Work out the finished part from the listing and answer in its coordinate system (mm). A direction names the side the tool comes from. Give positions to 0.01 mm unless a question says otherwise; leave off trailing zeros. Loops run counter-clockwise (first coordinate to the right, second up) from the corner with the lowest first, then second, coordinate; pieces in that order, holes last. Notation, with made-up numbers: (59, 6) -> (105, 6) arc R16 cw to (105, 34) -> close; hole circle Ø2 at (-4.75, -18.75). An arc over 180 degrees is marked (long way). Answer as CSV lines item,"result". Start each with the question number.
1. Flat-ended cylindrical pins translate along their axes: pin 1 Ø6.5 at (y, z) = (252, 0) entering from +X; pin 2 Ø3.5 at (y, z) = (10, 0) entering from +X; pin 3 Ø1.5 at (x, z) = (-3, 0) entering from -Y; pin 4 Ø1.5 at (x, y) = (-3, 196.5) entering from +Z. Find the tip coordinate at first contact, or state that the pin passes through.
2. Find section D-D, the plane y = 10. Give the vertices of the cut face in (x, z).
3. A tool of negligible diameter and unlimited length cuts with its end or side. For faces 4 (the face through (4.99, 7.97, 2.21)), 5 (the face through (-4.77, 128.18, -1.5)), from which of +Z, -Z, +X, -X, +Y, -Y can it reach the whole face along a straight path? Write none if from no direction.
4. Find the intervals of material crossed by line 1 along Z through (x, y) = (0, 143); line 2 along Z through (x, y) = (-0.75, 213), in increasing order.
5. Find section A-A, the plane z = 0. Give the vertices of the cut face in (x, y).
6. Determine the mould class of faces 1 (the face through (-5.723, 128.18, -1.802)), 2 (the face through (4, 260, 4)), 3 (the face through (5.281, 253.952, 0.434)) for opening direction Z: +Z half, -Z half, draft (parallel to the pull), parting line (faces both ways), or undercut.
7. Find section B-B, the plane x = 0. Give the vertices of the cut face in (y, z).
8. Find section C-C, the plane y = 84. Give the vertices of the cut face in (x, z), and give its area (3 significant figures).
Autodesk Inventor part; units mm, degrees
ref_plane "Work Plane3" through (6, 0, 0) normal (1, 0, 0) x (0, 1, 0)
ref_plane "XZ Plane" through (0, 0, 0) normal (0, 1, 0) x (-1, 0, 0)
ref_plane "XY Plane" through (0, 0, 0) normal (0, 0, 1) x (1, 0, 0)
sketch "Sketch1" plane through (0, 0, 0) normal (0, 1, 0) x (-1, 0, 0)
  circle A0 centre (0, 0) radius 5
  circle A1 centre (0, 0) radius 6
  dimension "d0" = 12
  dimension "d1" = 1
extrude "Extrusion1" add sketch "Sketch1" along normal blind 260
ref_plane "Work Plane3" through (6, 0, 0) normal (1, 0, 0) x (0, 1, 0)
sketch "Sketch2" plane through (6, 0, 0) normal (1, 0, 0) x (0, 1, 0)
  line L0 (0, -6) -> (260, -6)
  line L1 (0, 6) -> (260, 6)
  line L2 (260, -6) -> (260, 6)
  line L3 (-60, 0) -> (360, 0)
  point P0 (0, 0)
  point P1 (10, 0)
  point P2 (252, 0)
  point P3 (260, 0)
  dimension "d20" = 10
  dimension "d21" = 8
hole "Hole1" at (6, 10, 0) direction (-1, 0, 0) diameter 6 end up to surface
hole "Hole2" at (6, 252, 0) direction (-1, 0, 0) diameter 4 end up to surface
equation "\"d2\" = pipe_length"
equation "\"pipe_length\" = -hinge_arm_length + hinge_insertion - 0.5 * box_diameter + 0.5 * stand_diameter - connection_length - margin_for_connection"
equation "\"stand_diameter\" = 800"
equation "\"hinge_insertion\" = 15"
equation "\"connection_length\" = 20"
equation "\"box_diameter\" = 200"
equation "\"hinge_arm_length\" = 25"
equation "\"margin_for_connection\" = 10"
properties part number "pipe" material "Aluminum 6061"
Resolved:
1,pin 1,"stops at x = 6"
1,pin 2,"stops at x = -4.68"
1,pin 3,"passes through"
1,pin 4,"stops at z = 5.56"
2,outline,"(4, -3) arc R5 cw (long way) to (4, 3) -> (5.2, 3) arc R6 ccw (long way) to (5.2, -3) -> close"
3,face 4,"+X"
3,face 5,"+Y, -Y"
4,line 1,"z = -6 to -5, 5 to 6"
4,line 2,"z = -5.95 to -4.94, 4.94 to 5.95"
5,outline,"(-6, 0) -> (-5, 0) -> (-5, 260) -> (-6, 260) -> close; (5, 0) -> (6, 0) -> (6, 7) -> (5, 7) -> close; (5, 13) -> (6, 13) -> (6, 250) -> (5, 250) -> close; (5, 254) -> (6, 254) -> (6, 260) -> (5, 260) -> close"
6,face 1,"parting line"
6,face 2,"draft"
6,face 3,"undercut"
7,outline,"(0, -6) -> (260, -6) -> (260, -5) -> (0, -5) -> close; (0, 5) -> (260, 5) -> (260, 6) -> (0, 6) -> close"
8,outline,"circle Ø12 at (0, 0); hole circle Ø10 at (0, 0)"
8,area,"34.6 mm^2"
